Input: part model. Units: mm. Frame: model coordinates. Give positions to 0.01 mm unless a question says otherwise; leave off trailing zeros. Order: outer loops, then holes, each group sorted by start corner. A loop starts at its lowest first (then second) coordinate and runs counter-clockwise, first axis right, second up. Notation, with made-up numbers: (22.5, -40) -> (60.5, -40) arc R16 cw to (60.5, -15) -> close; hole circle Ø7 at (13, 40). An arc over 180 degrees is marked (long way). Use a Markdown table: item, result. Add a question column.
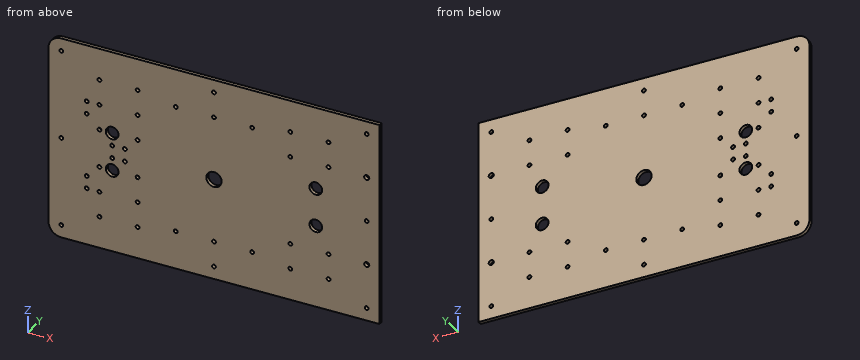
from build123d import *

# Parameters (mm, degrees)
SKETCH_1_W                 = 260
SKETCH_1_H                 = 160
EXTRUDE_1_DEPTH            = 3
SKETCH_2_R                 = 1.5
SKETCH_2_R_2               = 5
CUT_EXTRUDE_1_DEPTH        = 10
MIRROR_2_COPY_1_SKETCH_R   = 1.5
MIRROR_2_COPY_1_SKETCH_R_2 = 5
MIRROR_2_COPY_1_DEPTH      = 10
SKETCH_3_R                 = 6
CUT_EXTRUDE_2_DEPTH        = 10
SKETCH_4_R                 = 1.5
CUT_EXTRUDE_3_DEPTH        = 10
SKETCH_5_R                 = 1.5
CUT_EXTRUDE_4_DEPTH        = 10
FILLET_1_R                 = 10
SKETCH_6_R                 = 1.5
CUT_EXTRUDE_5_DEPTH        = 10
SKETCH_7_R                 = 1.5
CUT_EXTRUDE_6_DEPTH        = 10
SKETCH_8_R                 = 2
CUT_EXTRUDE_7_DEPTH        = 153.672852859


with BuildPart() as part:
    # 草图1 → 凸台-拉伸1 (new body)
    with BuildSketch(Plane(origin=(0, 0, 0), x_dir=(1, 0, 0), z_dir=(0, 1, 0))):
        Rectangle(SKETCH_1_W, SKETCH_1_H)
    extrude(amount=EXTRUDE_1_DEPTH)

    # 草图2 → 切除-拉伸1 (cut)
    with BuildSketch(Plane(origin=(0, 3, 0), x_dir=(1, 0, 0), z_dir=(0, 1, 0))):
        with Locations(Location((-90, 55, 0), (0, 0, 270))):
            Circle(SKETCH_2_R)
        with Locations(Location((-60, 55, 0), (0, 0, 270))):
            Circle(SKETCH_2_R)
        with Locations(Location((-90, 35, 0), (0, 0, 270))):
            Circle(SKETCH_2_R)
        with Locations(Location((-60, 35, 0), (0, 0, 270))):
            Circle(SKETCH_2_R)
        with Locations(Location((-80, 15, 0), (0, 0, 270))):
            Circle(SKETCH_2_R_2)
    cut_extrude_1 = extrude(amount=-CUT_EXTRUDE_1_DEPTH, mode=Mode.SUBTRACT)

    # 镜向1: 切除-拉伸1 across plane
    add(cut_extrude_1.mirror(Plane.XY), mode=Mode.SUBTRACT)

    # 镜向2: 切除-拉伸1 across plane
    add(cut_extrude_1.mirror(Plane(origin=(0, 0, 0), x_dir=(0, 0, 1), z_dir=(1, 0, 0))), mode=Mode.SUBTRACT)

    # 镜向2 copy 1 sketch → 镜向2 copy 1 (cut)
    with BuildSketch(Plane(origin=(0, 3, 0), x_dir=(-1, 0, 0), z_dir=(0, 1, 0))):
        with Locations(Location((-90, 55, 0), (0, 0, 270))):
            Circle(MIRROR_2_COPY_1_SKETCH_R)
        with Locations(Location((-60, 55, 0), (0, 0, 270))):
            Circle(MIRROR_2_COPY_1_SKETCH_R)
        with Locations(Location((-90, 35, 0), (0, 0, 270))):
            Circle(MIRROR_2_COPY_1_SKETCH_R)
        with Locations(Location((-60, 35, 0), (0, 0, 270))):
            Circle(MIRROR_2_COPY_1_SKETCH_R)
        with Locations(Location((-80, 15, 0), (0, 0, 270))):
            Circle(MIRROR_2_COPY_1_SKETCH_R_2)
    extrude(amount=-MIRROR_2_COPY_1_DEPTH, mode=Mode.SUBTRACT)

    # 草图3 → 切除-拉伸2 (cut)
    with BuildSketch(Plane(origin=(0, 3, 0), x_dir=(1, 0, 0), z_dir=(0, 1, 0))):
        with Locations(Location((0, 0, 0), (0, 0, 270))):
            Circle(SKETCH_3_R)
    extrude(amount=-CUT_EXTRUDE_2_DEPTH, mode=Mode.SUBTRACT)

    # 草图4 → 切除-拉伸3 (cut)
    with BuildSketch(Plane.XZ):
        with Locations(Location((0, 50, 0), (0, 0, 270))):
            Circle(SKETCH_4_R)
        with Locations(Location((-30, 50, 0), (0, 0, 270))):
            Circle(SKETCH_4_R)
        with Locations(Location((30, 50, 0), (0, 0, 270))):
            Circle(SKETCH_4_R)
    cut_extrude_3 = extrude(amount=-CUT_EXTRUDE_3_DEPTH, mode=Mode.SUBTRACT)

    # 镜向3: 切除-拉伸3 across plane
    add(cut_extrude_3.mirror(Plane.XY), mode=Mode.SUBTRACT)

    # 草图5 → 切除-拉伸4 (cut)
    with BuildSketch(Plane(origin=(0, 3, 0), x_dir=(1, 0, 0), z_dir=(0, 1, 0))):
        with Locations(Location((-80, 5, 0), (0, 0, 270))):
            Circle(SKETCH_5_R)
        with Locations(Location((-70, 5, 0), (0, 0, 270))):
            Circle(SKETCH_5_R)
        with Locations(Location((-90, 15, 0), (0, 0, 270))):
            Circle(SKETCH_5_R)
        with Locations(Location((-60, 15, 0), (0, 0, 270))):
            Circle(SKETCH_5_R)
        with Locations(Location((-100, 25, 0), (0, 0, 270))):
            Circle(SKETCH_5_R)
        with Locations(Location((-100, 35, 0), (0, 0, 270))):
            Circle(SKETCH_5_R)
    cut_extrude_4 = extrude(amount=-CUT_EXTRUDE_4_DEPTH, mode=Mode.SUBTRACT)

    # 镜向4: 切除-拉伸4 across plane
    add(cut_extrude_4.mirror(Plane.XY), mode=Mode.SUBTRACT)

    # 圆角1
    fillet_1_edges = [part.edges().sort_by_distance(p)[0] for p in [
        (-130, 1.5, -80),
        (-130, 1.5, 80),
    ]]
    fillet(fillet_1_edges, radius=FILLET_1_R)

    # 草图6 → 切除-拉伸5 (cut)
    with BuildSketch(Plane(origin=(0, 3, 0), x_dir=(1, 0, 0), z_dir=(0, 1, 0))):
        with Locations(Location((-120, 70, 0), (0, 0, 270))):
            Circle(SKETCH_6_R)
        with Locations(Location((0, 70, 0), (0, 0, 270))):
            Circle(SKETCH_6_R)
        with Locations(Location((120, 70, 0), (0, 0, 270))):
            Circle(SKETCH_6_R)
    cut_extrude_5 = extrude(amount=-CUT_EXTRUDE_5_DEPTH, mode=Mode.SUBTRACT)

    # 镜向5: 切除-拉伸5 across plane
    add(cut_extrude_5.mirror(Plane.XY), mode=Mode.SUBTRACT)

    # 草图7 → 切除-拉伸6 (cut)
    with BuildSketch(Plane(origin=(0, 3, 0), x_dir=(1, 0, 0), z_dir=(0, 1, 0))):
        with Locations(Location((-120, 0, 0), (0, 0, 270))):
            Circle(SKETCH_7_R)
        with Locations(Location((120, 0, 0), (0, 0, 270))):
            Circle(SKETCH_7_R)
    extrude(amount=-CUT_EXTRUDE_6_DEPTH, mode=Mode.SUBTRACT)

    # 草图8 → 切除-拉伸7 (cut, through all)
    with BuildSketch(Plane(origin=(0, 0, 0), x_dir=(-1, 0, 0), z_dir=(0, -1, 0))):
        with Locations(Location((-120, 35, 0), (0, 0, 90))):
            Circle(SKETCH_8_R)
        with Locations(Location((-120, -35, 0), (0, 0, 90))):
            Circle(SKETCH_8_R)
    extrude(amount=-CUT_EXTRUDE_7_DEPTH, mode=Mode.SUBTRACT)


solid = part.part
Q1. Section query A-A (x = 80). Return loops of the section in (y, z), plus the area to 3 significant figures.
Q2. First-contact query: pin 1 (2.5 mm diameter, centred on x = 0, z = -50, fed in from -Y). Flat tip, straight axial feed; report the tip coordinate or a pass-through.
Q3. Ray query, line 1 (Z direction, x = 60, y = 2.3); line 2 (X direction, y = 1.7, z = 0); line 3 (X direction, y = 1.6, z = 70). Return the intervals inside material, ascending.
Q4. Section query B-B (y = 2.45). Give the number of separate pieces and of enclosed holes in the cut face, plus the area to 3 significant figures.
Solution:
| question | item | result |
|---|---|---|
| 1 | outline | (0, -80) -> (3, -80) -> (3, -20) -> (0, -20) -> close; (0, -10) -> (3, -10) -> (3, 10) -> (0, 10) -> close; (0, 20) -> (3, 20) -> (3, 80) -> (0, 80) -> close |
| 1 | area | 420 mm² |
| 2 | pin 1 | passes through |
| 3 | line 1 | z = -80 to -56.5, -53.5 to -36.5, -33.5 to 33.5, 36.5 to 53.5, 56.5 to 80 |
| 3 | line 2 | x = -130 to -121.5, -118.5 to -6, 6 to 118.5, 121.5 to 130 |
| 3 | line 3 | x = -130 to -121.5, -118.5 to -1.5, 1.5 to 118.5, 121.5 to 130 |
| 4 | separate pieces | 1 |
| 4 | enclosed holes | 49 |
| 4 | area | 40,800 mm² |
